Study the drawing (mm; zero at the part's minimum x, y, z) and answer. Round coordinates to 2 decimals unless told otherwise and drop trailing zeros. Write each loop counter-clockwise with the first axis right and the second up, starting at its lowest first coordinate (ties: lowest second). Pieces come first, ordered by that corner, then holes. Notation, with made-up numbers: (-35.5, -35.75) - (-10.5, -35.75) arc R22 ccw to (-10.5, -26.75) - close; hole circle Ø9 at (15, -25.75). An arc over 180 degrees is marked (long way). Return JSON: item names as keys, results as strings. Group by question number.
(1) Find the intervals of material crossed by line 1 along X through (y, z) = (4.45, 31); line 2 along Z through (x, y) = (148, 1.7); line 3 along X through (y, z) = (3.6, 120), in increasing order. Write a range as [from, to].
(2) Section B-B, the plane x = 142.5 is taken. Write down the section's boundary in (y, z).
(3) Section A-A, the plane z = 87.5 is taken. Write down the section's boundary in (x, y).
(4) Each of these flat-tipped pins is pushed along its axis until it touches: pin 1 (2 mm diameter, centred on y = 4, z = 70.5, fed in from +X); pin 2 (2.5 mm diameter, centred on x = 76, y = 2, fed in from +Z); pin 3 (1.4 mm diameter, centred on x = 78, y = 3, fed in from -Z). Where does it stop, or does it pass through?
(5) Section D-D, the plane x = 78 is taken. Write down the section's boundary in (y, z).
(6) Section C-C, the plane y = 2.7 is taken. Write down the section's boundary in (x, z).
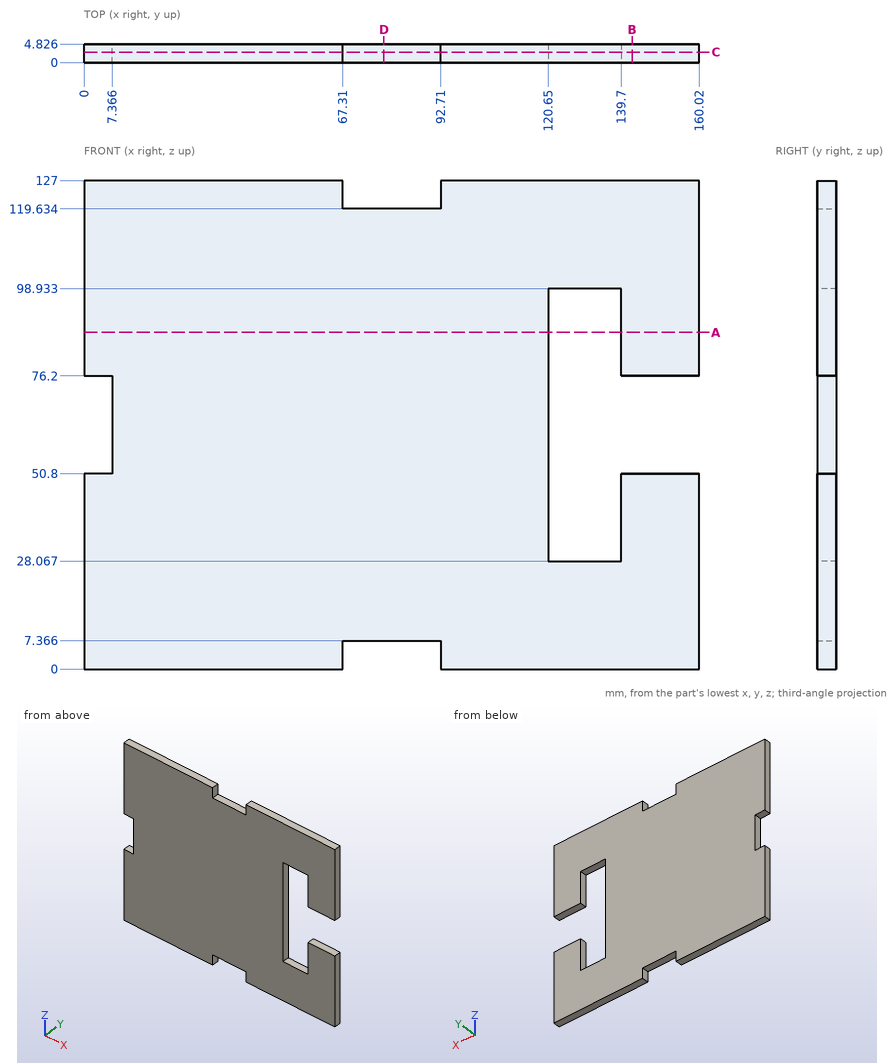
Working result:
{
 "1": {"line 1": "x = [0, 120.65], [139.7, 160.02]", "line 2": "z = [0, 50.8], [76.2, 127]", "line 3": "x = [0, 67.31], [92.71, 160.02]"},
 "2": {"outline": "(0, 0) - (4.83, 0) - (4.83, 50.8) - (0, 50.8) - close; (0, 76.2) - (4.83, 76.2) - (4.83, 127) - (0, 127) - close"},
 "3": {"outline": "(0, 0) - (120.65, 0) - (120.65, 4.83) - (0, 4.83) - close; (139.7, 0) - (160.02, 0) - (160.02, 4.83) - (139.7, 4.83) - close"},
 "4": {"pin 1": "stops at x = 120.65", "pin 2": "stops at z = 119.63", "pin 3": "stops at z = 7.37"},
 "5": {"outline": "(0, 7.37) - (4.83, 7.37) - (4.83, 119.63) - (0, 119.63) - close"},
 "6": {"outline": "(0, 0) - (67.31, 0) - (67.31, 7.37) - (92.71, 7.37) - (92.71, 0) - (160.02, 0) - (160.02, 50.8) - (139.7, 50.8) - (139.7, 28.07) - (120.65, 28.07) - (120.65, 98.93) - (139.7, 98.93) - (139.7, 76.2) - (160.02, 76.2) - (160.02, 127) - (92.71, 127) - (92.71, 119.63) - (67.31, 119.63) - (67.31, 127) - (0, 127) - (0, 76.2) - (7.37, 76.2) - (7.37, 50.8) - (0, 50.8) - close"}
}
